Could you check a few things on this model? Use its own coordinates, in mm. Face numbers are marked on the shaded views. A direction names the side the tool comes from. Coordinates: 2 decimals unless noted, no trailing zeros. Order: outer loops, then holes, each group sorted by start corner. A loop starts at its lowest first (then second) coordinate and runs counter-clockwise, first axis right, second up. Notation, with made-up numbers: (82.5, 37.5) - (91.5, 37.5) arc R11 cw to (91.5, 54.5) - close; hole circle Ø11 at (-28, -35). An arc over 180 degrees is marked (long way). One line per item, written item: value.
from build123d import *

# Parameters (mm, degrees)
SKETCH_2_R      = 2.6
SKETCH_2_R_2    = 3.9
EXTRUDE_1_DEPTH = 3.7
SKETCH_3_R      = 12.7
SKETCH_3_R_2    = 3.9
EXTRUDE_2_DEPTH = 5
SKETCH_4_R      = 6
SKETCH_4_R_2    = 3.9
EXTRUDE_3_DEPTH = 4.5


with BuildPart() as part:
    # 草圖2 → 填料-伸長1 (new body)
    with BuildSketch(Plane.XY):
        with BuildLine():
            Line((-20.181106134, 4.72046354), (-5.347916667, 11.574207849))
            ThreePointArc((-5.347916667, 11.574207849), (0, 12.75), (5.347916667, 11.574207849))
            Line((5.347916667, 11.574207849), (20.181106134, 4.72046354))
            ThreePointArc((20.181106134, 4.72046354), (23.2, 0), (20.181106134, -4.72046354))
            Line((20.181106134, -4.72046354), (5.347916667, -11.574207849))
            ThreePointArc((5.347916667, -11.574207849), (0, -12.75), (-5.347916667, -11.574207849))
            Line((-5.347916667, -11.574207849), (-20.181106134, -4.72046354))
            ThreePointArc((-20.181106134, -4.72046354), (-23.2, 0), (-20.181106134, 4.72046354))
        make_face()
        with Locations((-18, 0)):
            Circle(SKETCH_2_R, mode=Mode.SUBTRACT)
        with Locations((18, 0)):
            Circle(SKETCH_2_R, mode=Mode.SUBTRACT)
        Circle(SKETCH_2_R_2, mode=Mode.SUBTRACT)
    extrude(amount=EXTRUDE_1_DEPTH)

    # 草圖3 → 填料-伸長2 (add)
    with BuildSketch(Plane.XY.offset(3.7)):
        Circle(SKETCH_3_R)
        Circle(SKETCH_3_R_2, mode=Mode.SUBTRACT)
    extrude(amount=EXTRUDE_2_DEPTH)

    # 草圖4 → 填料-伸長3 (add)
    with BuildSketch(Plane.XY.offset(8.7)):
        Circle(SKETCH_4_R)
        Circle(SKETCH_4_R_2, mode=Mode.SUBTRACT)
    extrude(amount=EXTRUDE_3_DEPTH)


solid = part.part
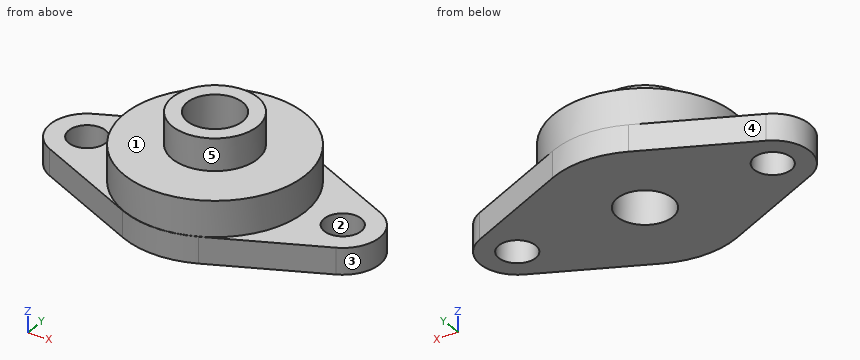
Item 1: I want a section at A-A on y = 0. Please give me the cut outline in (x, z), then the cut area to 3 significant figures.
Conclusion:
outline: (-23.2, 0) - (-20.6, 0) - (-20.6, 3.7) - (-23.2, 3.7) - close; (-15.4, 0) - (-3.9, 0) - (-3.9, 13.2) - (-6, 13.2) - (-6, 8.7) - (-12.7, 8.7) - (-12.7, 3.7) - (-15.4, 3.7) - close; (3.9, 0) - (15.4, 0) - (15.4, 3.7) - (12.7, 3.7) - (12.7, 8.7) - (6, 8.7) - (6, 13.2) - (3.9, 13.2) - close; (20.6, 0) - (23.2, 0) - (23.2, 3.7) - (20.6, 3.7) - close
area: 211 mm²
Item 2: For the marked faces 4 and 5, which set-ups out of +Z, -Z, +X, -X, +Y, -Y let a thin tool reach every point of the face, with its end or its side?
Conclusion:
face 4: +Z, -Z, -X, +Y
face 5: +Z
Item 3: I want a section at C-C on z = 3. Please give me the cut outline in (x, y).
Conclusion:
outline: (-20.18, -4.72) - (-5.35, -11.57) arc R12.75 ccw to (5.35, -11.57) - (20.18, -4.72) arc R5.2 ccw to (20.18, 4.72) - (5.35, 11.57) arc R12.75 ccw to (-5.35, 11.57) - (-20.18, 4.72) arc R5.2 ccw to start; hole circle Ø5.2 at (-18, 0); hole circle Ø7.8 at (0, 0); hole circle Ø5.2 at (18, 0)
Item 4: I'm going to push flat-ended pins straight in: pin 1 Ø4 at (y, z) = (1, 5.5) entering from -X; pin 2 Ø4 at (y, z) = (-10, 3) entering from +X; pin 3 Ø5 at (x, z) = (-4, 5.5) entering from +Y; pin 4 Ø3 at (x, y) = (18, 0) entering from -Z. Where does each tip first touch, or does it pass through?
Conclusion:
pin 1: x = -23.2
pin 2: x = 13.08
pin 3: y = 12.61
pin 4: through
Item 5: I want a section at D-D on x = -7. Please give me the cut outline in (y, z), then the cut area to 3 significant figures.
Conclusion:
outline: (-10.81, 0) - (10.81, 0) - (10.81, 3.7) - (10.6, 3.7) - (10.6, 8.7) - (-10.6, 8.7) - (-10.6, 3.7) - (-10.81, 3.7) - close
area: 186 mm²
Item 6: I want a section at B-B on x = 0. Please give me the cut outline in (y, z), then the cut area to 3 significant figures.
Conclusion:
outline: (-12.75, 0) - (-3.9, 0) - (-3.9, 13.2) - (-6, 13.2) - (-6, 8.7) - (-12.7, 8.7) - (-12.7, 3.7) - (-12.75, 3.7) - close; (3.9, 0) - (12.75, 0) - (12.75, 3.7) - (12.7, 3.7) - (12.7, 8.7) - (6, 8.7) - (6, 13.2) - (3.9, 13.2) - close
area: 172 mm²
Item 7: Thinking about a two-plate mould opening in X: for the marked faces 1, 2 and 3, which applies, pulls with the +X half, pulls with the -X half, needs draft (parallel to the pull), parting line crosses it, or undercut?
Conclusion:
face 1: needs draft
face 2: undercut
face 3: pulls with the +X half
Item 8: If I drill on probe 1 along Y at (x, z) = (0, 8); probe 2 along Y at (x, z) = (0, 10); probe 3 along Z at (x, y) = (16, 2.25), over which ranges is the centre line in solid material (lowest first)?
Conclusion:
probe 1: -12.7 to -3.9, 3.9 to 12.7
probe 2: -6 to -3.9, 3.9 to 6
probe 3: 0 to 3.7
